from build123d import *

# Parameters (mm, degrees)
BOSS_EXTRUDE1_DEPTH = 1.6
SKETCH2_R           = 2.1
CUT_EXTRUDE1_DEPTH  = 2.6
LPATTERN1_COUNT     = 11
LPATTERN1_PITCH     = 8


with BuildPart() as part:
    # Sketch1 → Boss-Extrude1 (new body)
    with BuildSketch(Plane(origin=(0, 0, 0), x_dir=(1, 0, 0), z_dir=(0, 1, 0))):
        with BuildLine():
            Line((4.85, 4.85), (83.15, 4.85))
            ThreePointArc((83.15, 4.85), (88, 0), (83.15, -4.85))
            Line((83.15, -4.85), (4.85, -4.85))
            ThreePointArc((4.85, -4.85), (0, 0), (4.85, 4.85))
        make_face()
    extrude(amount=BOSS_EXTRUDE1_DEPTH)

    # Sketch2 → Cut-Extrude1 (cut, through all)
    with BuildSketch(Plane(origin=(0, 1.6, 0), x_dir=(1, 0, 0), z_dir=(0, 1, 0))):
        with Locations((4, 0)):
            Circle(SKETCH2_R)
    cut_extrude1 = extrude(amount=-CUT_EXTRUDE1_DEPTH, mode=Mode.SUBTRACT)

    # LPattern1: Cut-Extrude1 ×11
    with Locations(*[(i * LPATTERN1_PITCH, 0, 0) for i in range(1, LPATTERN1_COUNT)]):
        add(cut_extrude1, mode=Mode.SUBTRACT)


solid = part.part
Build history of the part. All positions in model axes, mm. Give positions to 0.01 mm unless a question says otherwise; leave off trailing zeros. Loops run counter-clockwise (first coordinate to the right, second up) from the corner with the lowest first, then second, coordinate; pieces in that order, holes last. Notation, with made-up numbers: (49.25, 64.25) -> (72.25, 64.25) arc R32 cw to (72.25, 98.25) -> close; hole circle Ø5 at (43, 39.5). An arc over 180 degrees is marked (long way). Answer in a Markdown table with one row per item.
Item 1: Slice it at B-B on y = 0.9. Give the number of separate pieces and of enclosed holes in the cut face, plus the area to 3 significant figures.
Findings below:
| item | result |
|---|---|
| separate pieces | 1 |
| enclosed holes | 11 |
| area | 681 mm² |
Item 2: Slice it at D-D on x = 27.5. Write the cut outline in (y, z).
Findings below:
| item | result |
|---|---|
| outline | (0, -4.85) -> (1.6, -4.85) -> (1.6, -2.04) -> (0, -2.04) -> close; (0, 2.04) -> (1.6, 2.04) -> (1.6, 4.85) -> (0, 4.85) -> close |
Item 3: Mould opens along X. For faces 1 (the cylindrical face through (25.9, 0.81, -0.09)), 2 (the cylindrical face through (22.003, 0.811, -0.631)), 3 (the cylindrical face through (0, 1, 0)), 4 (the flat face through (43, 1, -4.85)) say: pulls with the +X half, pulls with the -X half, needs draft (parallel to the pull), parting line crosses it, or undercut.
Findings below:
| item | result |
|---|---|
| face 1 | undercut |
| face 2 | undercut |
| face 3 | pulls with the -X half |
| face 4 | needs draft |
Item 4: Flat gauge pin, fed straight in: P1, Ø3.5, axis at x = 4, z = 0, coming from the +Y side. Where does the tip first touch, or does it go through?
Findings below:
| item | result |
|---|---|
| P1 | passes through |
Item 5: Probe line 1 along Z through (x, y) = (20, 0.6); line 2 along Z through (x, y) = (53.5, 0.25); line 3 along X through (y, z) = (1.1, 2.5). List the from-to ranges inside material, lowest first. Write a range as [from, to].
Findings below:
| item | result |
|---|---|
| line 1 | z = [-4.85, -2.1], [2.1, 4.85] |
| line 2 | z = [-4.85, -1.47], [1.47, 4.85] |
| line 3 | x = [0.69, 87.31] |
Item 6: Slice it at A-A on x = 12. Write the cut outline in (y, z), plus the area to 3 significant figures.
Findings below:
| item | result |
|---|---|
| outline | (0, -4.85) -> (1.6, -4.85) -> (1.6, -2.1) -> (0, -2.1) -> close; (0, 2.1) -> (1.6, 2.1) -> (1.6, 4.85) -> (0, 4.85) -> close |
| area | 8.80 mm² |
